Model file for the job. Use its own axes, mm. A direction names the side the tool comes from. Coordinates: 2 decimals unless noted, no trailing zeros. Write each loop counter-clockwise with the first axis right and the second up, starting at its lowest first coordinate (ties: lowest second). Pieces come first, ordered by that corner, then holes.
Q1. Which spindle directions (+Z, -Z, +X, -X, +Y, -Y) get a long thin tool onto all of the face, cutting with end or side? Do faces 4 (the flat face through (3, 130.175, 391)), 5 (the flat face through (-3, -130.175, 82)), 6 (the flat face through (-3, 2, -4.762)). Say none if no direction does.
Q2. Band-saw the part on A-A, the plane x = 67.5. Write the cut outline in (y, z) (1 decimal).
Q3. Band-saw the part on B-B, the plane z = 73. Write the cut outline in (x, y) (3 decimals), plus the area to 3 significant figures.
Q4. Pin check, flat tips, straight feed: P1, Ø2, axis at x = -103.5, y = 47.5, coming from the +Z side; P2, Ø5, axis at x = -34, y = -135.5, coming from the +Z side; P3, Ø5, axis at x = -141.5, z = 566, coming from the -Y side (3 decimals); P4, Ø5.5, axis at y = 101.76, z = 42.31, coming from the +X side. Stop position of each tip, or through.
Q5. Band-saw the part on D-D, the plane y = -21. Write the cut outline in (x, z), plus the area to 3 significant figures.
Q6. Band-saw the part on C-C, the plane z = 327.5. Write the cut outline in (x, y) (3 decimals), plus the area to 3 significant figures.
Q7. Drill centre lines: probe 1 along Y at (x, z) = (195, 71.5) (3 decimals); probe 2 along Z at (x, y) = (169.5, 109.5); probe 3 along Y at (x, z) = (-37.5, 539) (3 decimals). Where is each one in solid material? Low to high.
Q8. Pull direction Y, two halves, no side cores. Call faces 1 (the flat face through (-231.775, 105.2, 46.2)), 2 (the flat face through (-3, -139.7, 77)), 3 (the flat face through (241.3, 135, 211)): released by +Y, released by -Y, zero draft, split by the parting line, or undercut.
from build123d import *

# Parameters (mm, degrees)
F0_W     = 482.6
F0_H     = 279.4
F1_DEPTH = 4.7625
F2_W     = 482.6
F2_H     = 762
F3_DEPTH = 9.525
F4_W     = 482.6
F4_H     = 152.4
F5_DEPTH = 9.525
F7_DEPTH = 9.525
F9_D     = 9.525


# Not quite as in the source:
# - a pattern or mirror of a feature is missing from the dataset's text; its kind, count and spacing are read off the source's solid


with BuildPart() as f1:
    # F0 (on Top) → F1 (new body, symmetric)
    with BuildSketch(Plane.XY):
        Rectangle(F0_W, F0_H)
    extrude(amount=F1_DEPTH, both=True)

    # F2 (on face) → F3 (join)
    with BuildSketch(Plane(origin=(0, 139.7, 0), x_dir=(-1, 0, 0), z_dir=(0, 1, 0))):
        with Locations((0, 385.7625)):
            Rectangle(F2_W, F2_H)
    extrude(amount=-F3_DEPTH)

    # F4 (on face) → F5 (join)
    with BuildSketch(Plane.XZ.offset(139.7)):
        with Locations((0, 80.9625)):
            Rectangle(F4_W, F4_H)
    extrude(amount=-F5_DEPTH)

    # F6 (on face) → F7 (join)
    with BuildSketch(Plane(origin=(-241.3, 0, 0), x_dir=(0, -1, 0), z_dir=(-1, 0, 0))):
        Polygon((-37.9520058632, 4.7625), (-130.175, 150.3834724426), (-130.175, 4.7625), align=None)
    f7 = extrude(amount=-F7_DEPTH)

    # F7_copies: F7 across plane
    add(f7.mirror(Plane(origin=(0, 0, 0), x_dir=(0, 0, 1), z_dir=(1, 0, 0))))

    # F9 (through all)
    with Locations(Plane.YZ.offset(241.3)):
        with Locations((101.7590165138, 42.3114337027)):
            Hole(F9_D / 2)


solid = f1.part
Answer sheet:
1. face 4: +Z
1. face 5: +Z, +X, -X
1. face 6: -Z, +X, -X, +Y, -Y
2. outline: (-139.7, -4.8) - (139.7, -4.8) - (139.7, 766.8) - (130.2, 766.8) - (130.2, 4.8) - (-130.2, 4.8) - (-130.2, 157.2) - (-139.7, 157.2) - close
3. outline: (-241.3, -139.7) - (241.3, -139.7) - (241.3, -130.175) - (-241.3, -130.175) - close; (-241.3, 81.167) - (-231.775, 81.167) - (-231.775, 130.175) - (231.775, 130.175) - (231.775, 81.167) - (241.3, 81.167) - (241.3, 139.7) - (-241.3, 139.7) - close
3. area: 10,100 mm2
4. P1: stops at z = 4.76
4. P2: stops at z = 157.16
4. P3: stops at y = 130.175
4. P4: passes through
5. outline: (-241.3, -4.76) - (241.3, -4.76) - (241.3, 4.76) - (-241.3, 4.76) - close
5. area: 4,600 mm2
6. outline: (-241.3, 130.175) - (241.3, 130.175) - (241.3, 139.7) - (-241.3, 139.7) - close
6. area: 4,600 mm2
7. probe 1: y = -139.7 to -130.175, 130.175 to 139.7
7. probe 2: z = -4.76 to 4.76
7. probe 3: y = 130.175 to 139.7
8. face 1: undercut
8. face 2: released by -Y
8. face 3: zero draft
